Read the model definition and answer for the solid it produces. Units are mm, in the model's axes. Face numbers are marked on the shaded views. A direction names the side the tool comes from. Round coordinates to 2 decimals unless told otherwise and drop trailing zeros. Write each loop counter-clockwise with the first axis right and the second up, starting at its lowest first coordinate (ties: lowest second). Pieces come first, ordered by that corner, then holes. Notation, with made-up numbers: (52, 23) - (111, 23) arc R6 ccw to (111, 30) - close; hole circle Ø3 at (-16.75, 64). An arc over 180 degrees is marked (long way). One line per item, written item: value. Start each with the question number.
(1) Flat-ended cylindrical pins translate along their axes: pin 1 Ø1 at (x, z) = (2, -2) entering from +Y; pin 2 Ø1 at (x, z) = (0.5, -2.5) entering from -Y; pin 3 Ø0.8 at (x, y) = (2, 2) entering from -Z. Find the tip coordinate at first contact, or state that the pin passes through.
(2) A cutting plane is placed at B-B, the plane z = -4.25. Determine the outline of the cut face in (x, y), plus the area to 3 significant figures.
(3) Find the intervals of material crossed by L1, parallel to X at y = 2, z = -10; L2, parallel to Z at x = 2, y = 2, in increasing order.
(4) The mould has two halves that part along Z. Classify the marked faces 1, 2 and 3: +Z half, -Z half, draft (parallel to the pull), parting line (faces both ways), or undercut.
(5) A cutting plane is placed at C-C, the plane x = 3. Determine the outline of the cut face in (y, z), plus the area to 3 significant figures.
(6) For the marked faces 4 and 5, determine the directions among +Z, -Z, +X, -X, +Y, -Y from which every point of the face is accessible in a straight line to the end or side of a thin tool.
(7) A cutting plane is placed at D-D, the plane y = 5. Determine the outline of the cut face in (x, z), plus the area to 3 significant figures.
(8) A cutting plane is placed at A-A, the plane y = 2. Determine the outline of the cut face in (x, z), plus the area to 3 significant figures.
from build123d import *

# Parameters (mm, degrees)
ESQUISSE4_W             = 8
ESQUISSE4_H             = 4
BOSS_EXTRU_2_DEPTH      = 4
ESQUISSE10_R            = 0.8
ENL_V_MAT_EXTRU_3_DEPTH = 8
ENL_V_START             = -4
ESQUISSE11_R            = 0.8
ENL_V_MAT_EXTRU_4_DEPTH = 4
ESQUISSE7_R             = 0.8
ENL_V_MAT_EXTRU_2_DEPTH = 8
CONG_4_R                = 2


with BuildPart() as part:
    # Esquisse4 → Boss.-Extru.2 (new body)
    with BuildSketch(Plane(origin=(0, 0, 0), x_dir=(0, 0, -1), z_dir=(1, 0, 0))):
        with Locations((8, 2)):
            Rectangle(ESQUISSE4_W, ESQUISSE4_H)
        Polygon((4, 0), (4, 4), (4, 12.5), (0, 12.5), (0, 0), align=None)
    extrude(amount=BOSS_EXTRU_2_DEPTH)

    # Esquisse10 → Enlèv. mat.-Extru.3 (cut)
    with BuildSketch(Plane(origin=(0, 12.5, 0), x_dir=(1, 0, 0), z_dir=(0, 1, 0))):
        with Locations(Location((2, 2, 0), (0, 0, 270))):
            Circle(ESQUISSE10_R)
    extrude(amount=-ENL_V_MAT_EXTRU_3_DEPTH, mode=Mode.SUBTRACT)

    # Esquisse11 → Enlèv. mat.-Extru.4 (cut)
    with BuildSketch(Plane.XZ.offset(ENL_V_START)):
        with Locations(Location((2, -2, 0), (0, 0, 90))):
            Circle(ESQUISSE11_R)
    extrude(amount=ENL_V_MAT_EXTRU_4_DEPTH, mode=Mode.SUBTRACT)

    # Esquisse7 → Enlèv. mat.-Extru.2 (cut)
    with BuildSketch(Plane(origin=(0, 0, -12), x_dir=(1, 0, 0), z_dir=(0, 0, -1))):
        with Locations(Location((2, -2, 0), (0, 0, 270))):
            Circle(ESQUISSE7_R)
    extrude(amount=-ENL_V_MAT_EXTRU_2_DEPTH, mode=Mode.SUBTRACT)

    # Congé4
    # the kernel refuses this fillet: 2 mm, written as the material it takes off along each edge
    with BuildSketch(Plane(origin=(4, 0, -17), x_dir=(-1, 0, 0), z_dir=(0, 0, 1)), Plane(origin=(0, 0, 5), x_dir=(1, 0, 0), z_dir=(0, 0, -1))) as cong_4_piece_1:
        with BuildLine():
            CenterArc((CONG_4_R, -CONG_4_R), CONG_4_R, 90, 90)
            Line((0, -CONG_4_R), (0, 0))
            Line((0, 0), (CONG_4_R, 0))
        make_face()
    extrude(amount=22, mode=Mode.SUBTRACT)
    with BuildSketch(Plane(origin=(4, 17.5, -4), x_dir=(0, 0, 1), z_dir=(0, -1, 0)), Plane(origin=(0, 4, -4), x_dir=(0, 0, 1), z_dir=(0, 1, 0))) as cong_4_piece_2:
        with BuildLine():
            CenterArc((CONG_4_R, CONG_4_R), CONG_4_R, 180, 90)
            Line((0, CONG_4_R), (0, 0))
            Line((0, 0), (CONG_4_R, 0))
        make_face()
    extrude(amount=13.5, mode=Mode.SUBTRACT)
    with BuildSketch(Plane(origin=(4, 4, -17), x_dir=(0, -1, 0), z_dir=(0, 0, 1))) as cong_4_piece_3:
        with BuildLine():
            CenterArc((CONG_4_R, -CONG_4_R), CONG_4_R, 90, 90)
            Line((0, -CONG_4_R), (0, 0))
            Line((0, 0), (CONG_4_R, 0))
        make_face()
    extrude(amount=13, mode=Mode.SUBTRACT)
    with BuildSketch(Plane(origin=(0, 4, -17), x_dir=(0, -1, 0), z_dir=(0, 0, 1))) as cong_4_piece_4:
        with BuildLine():
            CenterArc((CONG_4_R, CONG_4_R), CONG_4_R, 180, 90)
            Line((0, CONG_4_R), (0, 0))
            Line((0, 0), (CONG_4_R, 0))
        make_face()
    extrude(amount=13, mode=Mode.SUBTRACT)
    with BuildSketch(Plane(origin=(4, 17.5, 0), x_dir=(0, 0, -1), z_dir=(0, -1, 0))) as cong_4_piece_5:
        with BuildLine():
            CenterArc((CONG_4_R, -CONG_4_R), CONG_4_R, 90, 90)
            Line((0, -CONG_4_R), (0, 0))
            Line((0, 0), (CONG_4_R, 0))
        make_face()
    extrude(amount=22.5, mode=Mode.SUBTRACT)
    with BuildSketch(Plane(origin=(0, 17.5, 0), x_dir=(0, 0, -1), z_dir=(0, -1, 0))) as cong_4_piece_6:
        with BuildLine():
            CenterArc((CONG_4_R, CONG_4_R), CONG_4_R, 180, 90)
            Line((0, CONG_4_R), (0, 0))
            Line((0, 0), (CONG_4_R, 0))
        make_face()
    extrude(amount=22.5, mode=Mode.SUBTRACT)
    with BuildSketch(Plane(origin=(4, 4, -12), x_dir=(0, -1, 0), z_dir=(0, 0, 1))) as cong_4_piece_7a_section:
        with BuildLine():
            CenterArc((CONG_4_R, -CONG_4_R), CONG_4_R, 90, 90)
            Line((0, -CONG_4_R), (0, 0))
            Line((0, 0), (CONG_4_R, 0))
        make_face()
    cong_4_piece_7a = extrude(amount=13, mode=Mode.PRIVATE)
    cong_4_piece_7a = split(cong_4_piece_7a, bisect_by=Plane(origin=(4, 4, 0), z_dir=(0, 0, -1)), keep=Keep.TOP, mode=Mode.PRIVATE)
    cong_4_piece_7a = cong_4_piece_7a - Plane(origin=(2, 4, -2), x_dir=(0, 0, 1), z_dir=(0, 1, 0)) * Cylinder(0.8, 35, mode=Mode.PRIVATE)
    cong_4_piece_7a = split(cong_4_piece_7a, bisect_by=Plane(origin=(4, 4, -4), z_dir=(0, 0, 1)), keep=Keep.TOP, mode=Mode.PRIVATE)
    with BuildSketch(Plane(origin=(4, 12.5, -4), x_dir=(0, 0, 1), z_dir=(0, -1, 0))) as cong_4_piece_7b_section:
        with BuildLine():
            CenterArc((CONG_4_R, CONG_4_R), CONG_4_R, 180, 90)
            Line((0, CONG_4_R), (0, 0))
            Line((0, 0), (CONG_4_R, 0))
        make_face()
    cong_4_piece_7b = extrude(amount=13.5, mode=Mode.PRIVATE)
    cong_4_piece_7b = split(cong_4_piece_7b, bisect_by=Plane(origin=(4, 0, -4), z_dir=(0, 1, 0)), keep=Keep.TOP, mode=Mode.PRIVATE)
    cong_4_piece_7b = split(cong_4_piece_7b, bisect_by=Plane(origin=(4, 4, -4), z_dir=(0, -1, 0)), keep=Keep.TOP, mode=Mode.PRIVATE)
    cong_4_piece_7b = cong_4_piece_7b - Plane(origin=(2, 2, -4), x_dir=(0, 1, 0), z_dir=(0, 0, -1)) * Cylinder(0.8, 35, mode=Mode.PRIVATE)
    cong_4_piece_7 = cong_4_piece_7a & cong_4_piece_7b
    add(cong_4_piece_7, mode=Mode.SUBTRACT)
    with BuildSketch(Plane(origin=(0, 4, -12), x_dir=(0, -1, 0), z_dir=(0, 0, 1))) as cong_4_piece_8a_section:
        with BuildLine():
            CenterArc((CONG_4_R, CONG_4_R), CONG_4_R, 180, 90)
            Line((0, CONG_4_R), (0, 0))
            Line((0, 0), (CONG_4_R, 0))
        make_face()
    cong_4_piece_8a = extrude(amount=13, mode=Mode.PRIVATE)
    cong_4_piece_8a = split(cong_4_piece_8a, bisect_by=Plane(origin=(0, 4, 0), z_dir=(0, 0, -1)), keep=Keep.TOP, mode=Mode.PRIVATE)
    cong_4_piece_8a = cong_4_piece_8a - Plane(origin=(2, 4, -2), x_dir=(0, 0, 1), z_dir=(0, 1, 0)) * Cylinder(0.8, 35, mode=Mode.PRIVATE)
    cong_4_piece_8a = split(cong_4_piece_8a, bisect_by=Plane(origin=(0, 4, -4), z_dir=(0, 0, 1)), keep=Keep.TOP, mode=Mode.PRIVATE)
    with BuildSketch(Plane(origin=(0, -1, -4), x_dir=(0, 0, 1), z_dir=(0, 1, 0))) as cong_4_piece_8b_section:
        with BuildLine():
            CenterArc((CONG_4_R, CONG_4_R), CONG_4_R, 180, 90)
            Line((0, CONG_4_R), (0, 0))
            Line((0, 0), (CONG_4_R, 0))
        make_face()
    cong_4_piece_8b = extrude(amount=13.5, mode=Mode.PRIVATE)
    cong_4_piece_8b = split(cong_4_piece_8b, bisect_by=Plane(origin=(0, 0, -4), z_dir=(0, 1, 0)), keep=Keep.TOP, mode=Mode.PRIVATE)
    cong_4_piece_8b = split(cong_4_piece_8b, bisect_by=Plane(origin=(0, 4, -4), z_dir=(0, -1, 0)), keep=Keep.TOP, mode=Mode.PRIVATE)
    cong_4_piece_8b = cong_4_piece_8b - Plane(origin=(2, 2, -4), x_dir=(0, 1, 0), z_dir=(0, 0, -1)) * Cylinder(0.8, 35, mode=Mode.PRIVATE)
    cong_4_piece_8 = cong_4_piece_8a & cong_4_piece_8b
    add(cong_4_piece_8, mode=Mode.SUBTRACT)


solid = part.part
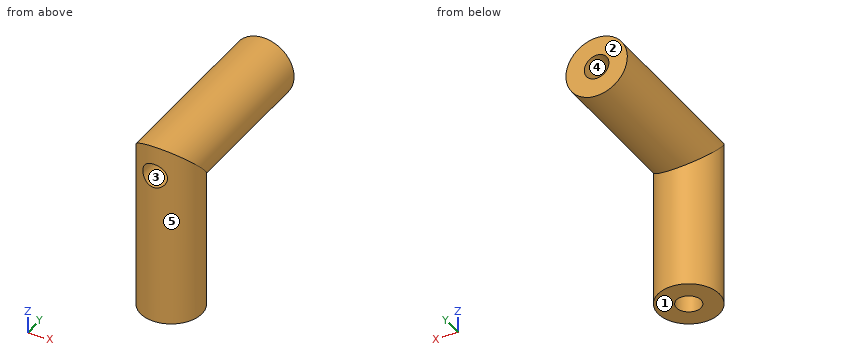
Here are the results:
1. pin 1: y = 4.5
1. pin 2: y = 0.27
1. pin 3: z = -4
2. outline: circle Ø4 at (2, 2); hole circle Ø1.6 at (2, 2)
2. area: 10.6 mm²
3. L1: 0 to 1.2, 2.8 to 4
3. L2: -4 to -2.8, -1.2 to 0
4. face 1: -Z half
4. face 2: draft
4. face 3: undercut
5. outline: (0.27, -12) - (3.73, -12) - (3.73, -3.73) - (12.5, -3.73) - (12.5, -0.27) - (0.27, -0.27) - close
5. area: 71.0 mm²
6. face 4: +Y
6. face 5: -Z
7. outline: circle Ø4 at (2, -2); hole circle Ø1.6 at (2, -2)
7. area: 10.6 mm²
8. outline: (0, -12) - (1.2, -12) - (1.2, -4) - (2.8, -4) - (2.8, -12) - (4, -12) - (4, -2) arc R2 ccw to (0, -2) - close; hole circle Ø1.6 at (2, -2)
8. area: 31.5 mm²
